```python
from build123d import *
from build123d.topology import SkipClean

# Parameters (mm, degrees)
BOSS_EXTRUDE1_DEPTH     = 27
BOSS_EXTRUDE2_DEPTH     = 65
CUT_EXTRUDE1_DEPTH      = 91.890043459
FILLET1_R               = 1
BOSS_EXTRUDE3_REACH     = 104.243
CUT_EXTRUDE2_REACH      = 104.243
BOSS_EXTRUDE4_REACH     = 92.026
BOSS_EXTRUDE5_DEPTH     = 65
SKETCH14_R              = 1.5
CUT_EXTRUDE7_DEPTH      = 5
CUT_EXTRUDE9_DEPTH      = 105.630301538
CUT_EXTRUDE9_DEPTH_BACK = 105.630301538
SKETCH15_W              = 45
SKETCH15_H              = 5.74
SKETCH16_R              = 1.5
CUT_EXTRUDE10_DEPTH     = 10
FILLET4_R               = 23
BOSS_EXTRUDE7_REACH     = 219.626
CUT_EXTRUDE5_DEPTH      = 184.620949427
CUT_EXTRUDE5_DEPTH_BACK = 184.620949427
SKETCH11_R              = 2.5
CUT_EXTRUDE6_DEPTH      = 186.847147779
CUT_EXTRUDE6_DEPTH_BACK = 186.847147779
SKETCH12_R              = 2.5
CUT_SWEEP1_START        = -43.471641414
CUT_SWEEP1_DEPTH        = 207.679031883


# Read off the part's stored shape, not the designer's step: Cut-Sweep1
with BuildPart() as part:
    # Sketch1 → Boss-Extrude1 (new body)
    with BuildSketch(Plane.XY):
        with BuildLine():
            Line((0, 0), (0, -26))
            ThreePointArc((0, -26), (32.5, -29.41402025), (65, -26))
            Line((65, -26), (65, 0))
            ThreePointArc((65, 0), (32.5, -3.41402025), (0, 0))
        make_face()
    extrude(amount=BOSS_EXTRUDE1_DEPTH)

    # Sketch4 → Boss-Extrude2 (add)
    with BuildSketch(Plane(origin=(65, 0, 0), x_dir=(0, 0, -1), z_dir=(1, 0, 0))):
        Polygon((0, -26), (30, -56), (30, -30), (0, 0), align=None)
    extrude(amount=-BOSS_EXTRUDE2_DEPTH)

    # Sketch5 → Cut-Extrude1 (cut, through all)
    with BuildSketch(Plane.XY):
        with BuildLine():
            Line((65, 0), (0, 0))
            ThreePointArc((0, 0), (32.5, -3.41402025), (65, 0))
        make_face()
    extrude(amount=-CUT_EXTRUDE1_DEPTH, mode=Mode.SUBTRACT)

    # Fillet1
    fillet1_edges = [part.edges().sort_by_distance(p)[0] for p in [
        (32.5, -56, -30),
    ]]
    fillet(fillet1_edges, radius=FILLET1_R)

    # Boss-Extrude3: up to this face of the body (flat: up to its plane)
    boss_extrude3_end = Plane(part.part.faces().sort_by_distance((32.5, -41.792893219, -30))[0])
    # Sketch6 → Boss-Extrude3 (add, up to the picked face)
    with BuildSketch(Plane.XY.offset(27), mode=Mode.PRIVATE) as boss_extrude3_sk1:
        with BuildLine():
            ThreePointArc((0, -26), (4.985486693, -26.974767058), (10, -27.787112227))
            Line((10, -27.787112227), (10, -1.787112227))
            ThreePointArc((10, -1.787112227), (4.985486693, -0.974767058), (0, 0))
            Line((0, 0), (0, -26))
        make_face()
    boss_extrude3_tool1 = split(extrude(boss_extrude3_sk1.sketch, amount=-BOSS_EXTRUDE3_REACH, mode=Mode.PRIVATE), bisect_by=boss_extrude3_end, keep=Keep.BOTH, mode=Mode.PRIVATE)
    # Sketch6 → Boss-Extrude3 (add, up to the picked face)
    with BuildSketch(Plane.XY.offset(27), mode=Mode.PRIVATE) as boss_extrude3_sk2:
        with BuildLine():
            Line((55, -1.787112227), (55, -27.787112227))
            ThreePointArc((55, -27.787112227), (60.014513307, -26.974767058), (65, -26))
            Line((65, -26), (65, 0))
            ThreePointArc((65, 0), (60.014513307, -0.974767058), (55, -1.787112227))
        make_face()
    boss_extrude3_tool2 = split(extrude(boss_extrude3_sk2.sketch, amount=-BOSS_EXTRUDE3_REACH, mode=Mode.PRIVATE), bisect_by=boss_extrude3_end, keep=Keep.BOTH, mode=Mode.PRIVATE)
    # Sketch6 → Boss-Extrude3 (add, up to the picked face)
    with BuildSketch(Plane.XY.offset(27), mode=Mode.PRIVATE) as boss_extrude3_sk3:
        with BuildLine():
            Line((10, -54.292893219), (10, -27.787112227))
            ThreePointArc((10, -27.787112227), (4.985486693, -26.974767058), (0, -26))
            Line((0, -26), (0, -54.292893219))
            Line((0, -54.292893219), (10, -54.292893219))
        make_face()
    boss_extrude3_tool3 = split(extrude(boss_extrude3_sk3.sketch, amount=-BOSS_EXTRUDE3_REACH, mode=Mode.PRIVATE), bisect_by=boss_extrude3_end, keep=Keep.BOTH, mode=Mode.PRIVATE)
    # Sketch6 → Boss-Extrude3 (add, up to the picked face)
    with BuildSketch(Plane.XY.offset(27), mode=Mode.PRIVATE) as boss_extrude3_sk4:
        with BuildLine():
            ThreePointArc((65, -26), (60.014513307, -26.974767058), (55, -27.787112227))
            Line((55, -27.787112227), (55, -54.292893219))
            Line((55, -54.292893219), (65, -54.292893219))
            Line((65, -54.292893219), (65, -26))
        make_face()
    boss_extrude3_tool4 = split(extrude(boss_extrude3_sk4.sketch, amount=-BOSS_EXTRUDE3_REACH, mode=Mode.PRIVATE), bisect_by=boss_extrude3_end, keep=Keep.BOTH, mode=Mode.PRIVATE)
    add(boss_extrude3_tool1.solids().sort_by(Axis((5, -13.949429, 27), (0, 0, -1)))[0])
    add(boss_extrude3_tool2.solids().sort_by(Axis((60, -13.949429, 27), (0, 0, -1)))[0])
    add(boss_extrude3_tool3.solids().sort_by(Axis((4.945547, -40.616285, 27), (0, 0, -1)))[0])
    add(boss_extrude3_tool4.solids().sort_by(Axis((60.054453, -40.616285, 27), (0, 0, -1)))[0])

    # Cut-Extrude2: up to this plane
    cut_extrude2_end = Plane(origin=(-63.529520697, -13, 13), z_dir=(0, -0.7071067811865562, 0.7071067811865389))
    # Sketch7 → Cut-Extrude2 (cut, up to the surface)
    with BuildSketch(Plane.XY.offset(27), mode=Mode.PRIVATE) as cut_extrude2_sk1:
        with BuildLine():
            ThreePointArc((10, -27.787112227), (4.985486693, -26.974767058), (0, -26))
            Line((0, -26), (0, -54.292893219))
            Line((0, -54.292893219), (10, -54.292893219))
            Line((10, -54.292893219), (10, -27.787112227))
        make_face()
    cut_extrude2_tool1 = split(extrude(cut_extrude2_sk1.sketch, amount=-CUT_EXTRUDE2_REACH, mode=Mode.PRIVATE), bisect_by=cut_extrude2_end, keep=Keep.BOTH, mode=Mode.PRIVATE)
    add(cut_extrude2_tool1.solids().sort_by_distance((4.945547, -40.616285, 27))[0], mode=Mode.SUBTRACT)
    # Sketch7 → Cut-Extrude2 (cut, up to the surface)
    with BuildSketch(Plane.XY.offset(27), mode=Mode.PRIVATE) as cut_extrude2_sk2:
        with BuildLine():
            Line((65, -54.292893219), (65, -26))
            ThreePointArc((65, -26), (60.014513307, -26.974767058), (55, -27.787112227))
            Line((55, -27.787112227), (55, -54.292893219))
            Line((55, -54.292893219), (65, -54.292893219))
        make_face()
    cut_extrude2_tool2 = split(extrude(cut_extrude2_sk2.sketch, amount=-CUT_EXTRUDE2_REACH, mode=Mode.PRIVATE), bisect_by=cut_extrude2_end, keep=Keep.BOTH, mode=Mode.PRIVATE)
    add(cut_extrude2_tool2.solids().sort_by_distance((60.054453, -40.616285, 27))[0], mode=Mode.SUBTRACT)

    # Boss-Extrude4: up to this face of the body (flat: up to its plane)
    boss_extrude4_end = Plane(part.part.faces().sort_by_distance((32.5, -40.28761869, -14.28761869))[0])
    # Sketch8 → Boss-Extrude4 (add, up to the picked face)
    with BuildSketch(Plane(origin=(0, 0, 0), x_dir=(-1, 0, 0), z_dir=(0, 0, -1)), mode=Mode.PRIVATE) as boss_extrude4_sk1:
        with BuildLine():
            Line((-55, -26), (-55, -27.787112227))
            ThreePointArc((-55, -27.787112227), (-32.5, -29.41402025), (-10, -27.787112227))
            Line((-10, -27.787112227), (-10, -26))
            Line((-10, -26), (-55, -26))
        make_face()
    boss_extrude4_tool1 = split(extrude(boss_extrude4_sk1.sketch, amount=BOSS_EXTRUDE4_REACH, mode=Mode.PRIVATE), bisect_by=boss_extrude4_end, keep=Keep.BOTH, mode=Mode.PRIVATE)
    add(boss_extrude4_tool1.solids().sort_by(Axis((32.5, -27.477312, 0), (0, 0, -1)))[0])

    # Sketch9 → Boss-Extrude5 (add)
    with BuildSketch(Plane.ZY):
        Polygon((-30, -51), (-25, -51), (-30, -56), align=None)
    extrude(amount=-BOSS_EXTRUDE5_DEPTH)

    # Sketch14 → Cut-Extrude7 (cut)
    with SkipClean():  # the faces are left unmerged after this step: merging them gives an invalid solid
        with BuildSketch(Plane(origin=(0, 0, 0), x_dir=(1, 0, 0), z_dir=(0, 0.7071067811865561, -0.7071067811865389))):
            with Locations(Location((14, 35.887280306, 0), (0, 0, 270))):
                Circle(SKETCH14_R)
            with Locations(Location((51, 35.887280306, 0), (0, 0, 270))):
                Circle(SKETCH14_R)
            with Locations(Location((51, 11.367280306, 0), (0, 0, 90))):
                Circle(SKETCH14_R)
            with Locations(Location((14, 11.367280306, 0), (0, 0, 90))):
                Circle(SKETCH14_R)
        extrude(amount=-CUT_EXTRUDE7_DEPTH, mode=Mode.SUBTRACT)

    # Sketch15 → Cut-Extrude9 (cut, two sides: drawn at the far end of the back side and taken through both)
    with SkipClean():  # the faces are left unmerged after this step: merging them gives an invalid solid
        with BuildSketch(Plane(origin=(0, 13.5, 13.5), x_dir=(-1, 0, 0), z_dir=(0, -0.7071067811865389, -0.7071067811865561)).offset(-CUT_EXTRUDE9_DEPTH_BACK)):
            with Locations((-32.5, -2.87)):
                Rectangle(SKETCH15_W, SKETCH15_H)
        extrude(amount=CUT_EXTRUDE9_DEPTH + CUT_EXTRUDE9_DEPTH_BACK, mode=Mode.SUBTRACT)

    # Sketch16 → Cut-Extrude10 (cut)
    with SkipClean():  # the faces are left unmerged after this step: merging them gives an invalid solid
        with BuildSketch(Plane(origin=(0, -4.058792924, 4.058792924), x_dir=(1, 0, 0), z_dir=(0, 0.7071067811865562, -0.7071067811865389))):
            with Locations(Location((14, 35.936406871, 0), (0, 0, 270))):
                Circle(SKETCH16_R)
            with Locations(Location((51, 35.936406871, 0), (0, 0, 270))):
                Circle(SKETCH16_R)
            with Locations(Location((14, 11.409221552, 0), (0, 0, 270))):
                Circle(SKETCH16_R)
            with Locations(Location((51, 11.409221552, 0), (0, 0, 270))):
                Circle(SKETCH16_R)
        extrude(amount=-CUT_EXTRUDE10_DEPTH, mode=Mode.SUBTRACT)

    # Fillet4
    fillet4_edges = [part.edges().sort_by_distance(p)[0] for p in [
        (32.5, -29.41402025, -3.41402025),
    ]]
    fillet(fillet4_edges, radius=FILLET4_R)

    # Boss-Extrude7: up to this face of the body (flat: up to its plane)
    boss_extrude7_end = Plane(part.part.faces().sort_by_distance((32.499999985, -45.563204914, -19.563204914))[0])
    # Sketch24 → Boss-Extrude7 (add, up to the picked face)
    with BuildSketch(Plane.XY.offset(170), mode=Mode.PRIVATE) as boss_extrude7_sk1:
        with BuildLine():
            Line((65, -56), (65, 0))
            ThreePointArc((65, 0), (60.014513307, -0.974767058), (55, -1.787112227))
            ThreePointArc((55, -1.787112227), (32.5, -3.41402025), (10, -1.787112227))
            ThreePointArc((10, -1.787112227), (4.985486693, -0.974767058), (0, 0))
            Line((0, 0), (0, -56))
            Line((0, -56), (65, -56))
        make_face()
    boss_extrude7_tool1 = split(extrude(boss_extrude7_sk1.sketch, amount=-BOSS_EXTRUDE7_REACH, mode=Mode.PRIVATE), bisect_by=boss_extrude7_end, keep=Keep.BOTH, mode=Mode.PRIVATE)
    add(boss_extrude7_tool1.solids().sort_by(Axis((32.5, -29.130902, 170), (0, 0, -1)))[0])

    # Sketch11 → Cut-Extrude5 (cut, two sides: drawn at the far end of the back side and taken through both)
    with BuildSketch(Plane(origin=(5.094217018, -35.042120851, 0), x_dir=(-0.9895977747865052, -0.14386189258312035, 0), z_dir=(-0.14386189258312035, 0.9895977747865053, 0)).offset(-CUT_EXTRUDE5_DEPTH_BACK)):
        with Locations(Location((-50.687468406, 22, 0), (0, 0, 180))):
            Circle(SKETCH11_R)
        with Locations(Location((-50.687468406, 147, 0), (0, 0, 180))):
            Circle(SKETCH11_R)
    extrude(amount=CUT_EXTRUDE5_DEPTH + CUT_EXTRUDE5_DEPTH_BACK, mode=Mode.SUBTRACT)

    # Sketch12 → Cut-Extrude6 (cut, two sides: drawn at the far end of the back side and taken through both)
    with BuildSketch(Plane(origin=(-3.74896115, -25.788369281, 0), x_dir=(0.9895977747865055, -0.14386189258311885, 0), z_dir=(-0.14386189258311885, -0.9895977747865056, 0)).offset(-CUT_EXTRUDE6_DEPTH_BACK)):
        with Locations(Location((13.636386955, 22, 0), (0, 0, 180))):
            Circle(SKETCH12_R)
        with Locations(Location((13.636386955, 147, 0), (0, 0, 180))):
            Circle(SKETCH12_R)
    extrude(amount=CUT_EXTRUDE6_DEPTH + CUT_EXTRUDE6_DEPTH_BACK, mode=Mode.SUBTRACT)

    # Cut-Sweep1 outline → Cut-Sweep1 (cut)
    with BuildSketch(Plane(origin=(0, 0, 0), x_dir=(1, 0, 0), z_dir=(0, 0.2588190451025179, 0.9659258262890691)).offset(CUT_SWEEP1_START)):
        with BuildLine():
            Line((65, -100), (65, -43.999237667))
            add(Edge.make_bspline(
                [(65, -43.999237667), (43.493313707, -48.412390901), (21.506686293, -48.412390901), (0, -43.999237667)],
                knots=[0, 0, 0, 0, 1, 1, 1, 1], degree=3, weights=[1, 0.985447484, 0.985447484, 1]))
            Line((0, -43.999237667), (0, -100))
            Line((0, -100), (65, -100))
        make_face()
    extrude(amount=CUT_SWEEP1_DEPTH, mode=Mode.SUBTRACT)


solid = part.part
```
Design review of the part built by this model. Coordinates are the model's own, in mm. A direction names the side the tool comes from. Coordinates: 2 decimals unless noted, no trailing zeros. Use CSV: the item, a comma, the result in double quotes. Start each with the question number.
1) The part is to be moulded in two halves that separate along X. For faces 3 (the flat face through (32, -56, -29)), 4 (the cylindrical face through (49.536, -15.842, -0.753)), 5 (the flat face through (65, -15, 27)), 6 (the cylindrical face through (15.265, -32.386, -17.296)), say which applies: +X half, -X half, draft (parallel to the pull), parting line (faces both ways), or undercut.
2) Wall thickness on L1, parallel to X at y = -23, z = -16; L2, parallel to Y at x = 48, z = 155.5; L3, parallel to Y at x = 38.5, z = 11.5: over which ranges is each line inside the solid? List them lowest first. Write a range as from..to.
3) Tool access review of faces 1 (the cylindrical face through (10.95, -21.74, 19.52)), 2 (the flat face through (55, -12, -20)): name each direction out of +Z, -Z, +X, -X, +Y, -Y from which nothing blocks a thin tool from reaching the whole face with its end or side.
4) For pin 1 Ø12 at (x, z) = (58, 37) entering from -Y; pin 2 Ø12 at (x, y) = (42, -19) entering from -Z; pin 3 Ø5 at (x, y) = (32, -9.5) entering from -Z, all flat-tipped, find the tip position at first contact; note any pin that passes through.
5) Consider section A-A on y = -5.5. Give the number of separate pieces and of enclosed holes in the cut face, then the cut area to 3 significant figures.
Geometry says:
1,face 3,"draft"
1,face 4,"undercut"
1,face 5,"+X half"
1,face 6,"undercut"
2,L1,"0..10, 55..65"
2,L2,"-6.53..-2.64"
2,L3,"-45.77..-3.3"
3,face 1,"none"
3,face 2,"-Z, +Y"
4,pin 1,"y = -38.82"
4,pin 2,"z = -16.88"
4,pin 3,"z = -3.88"
5,separate pieces,"1"
5,enclosed holes,"4"
5,area,"10,700 mm^2"
